from build123d import *

# Parameters (mm, degrees)
SKETCH1_R            = 5.3
BOSS_EXTRUDE1_DEPTH  = 15
M6_CLEARANCE_HOLE1_D = 6.6
BOSS_EXTRUDE3_DEPTH  = 2
BOSS_EXTRUDE2_DEPTH  = 8
SKETCH6_R            = 2.25
CUT_EXTRUDE1_DEPTH   = 27.870888862


with BuildPart() as part:
    # Sketch1 → Boss-Extrude1 (new body, symmetric)
    with BuildSketch(Plane(origin=(0, 0, 0), x_dir=(0, 0, -1), z_dir=(1, 0, 0))):
        Polygon((0, 12.912507763), (-29.037071095, -21.692526033), (-26.738937766, -23.620888862), (-13.883185572, -8.3), (13.883185572, -8.3), (26.738937766, -23.620888862), (29.037071095, -21.692526033), align=None)
        Circle(SKETCH1_R, mode=Mode.SUBTRACT)
    extrude(amount=BOSS_EXTRUDE1_DEPTH, both=True)

    # M6 Clearance Hole1 (through all)
    with Locations(Plane(origin=(0, 3.406774331, 4.060035549), x_dir=(-1, 0, 0), z_dir=(0, -0.64278761, -0.766044443))):
        with Locations((0, -25.282108547)):
            m6_clearance_hole1 = Hole(M6_CLEARANCE_HOLE1_D / 2)

    # Mirror1: M6 Clearance Hole1 across plane
    add(m6_clearance_hole1.mirror(Plane.XY), mode=Mode.SUBTRACT)

    # Sketch7 → Boss-Extrude3 (add)
    with BuildSketch(Plane.ZY.offset(15)):
        with BuildLine():
            Line((-5.150485414, 1.25), (-7.192183257, 1.25))
            ThreePointArc((-7.192183257, 1.25), (7.3, 0), (-7.192183257, -1.25))
            Line((-7.192183257, -1.25), (-5.150485414, -1.25))
            ThreePointArc((-5.150485414, -1.25), (5.3, 0), (-5.150485414, 1.25))
        make_face()
    extrude(amount=BOSS_EXTRUDE3_DEPTH)

    # Sketch5 → Boss-Extrude2 (add)
    with BuildSketch(Plane.ZY.offset(17)):
        with BuildLine():
            Line((-5.150485414, 1.25), (-14.536627571, 1.25))
            Line((-14.536627571, 1.25), (-14.536627571, 3.25))
            Line((-14.536627571, 3.25), (-6.536627571, 3.25))
            ThreePointArc((-6.536627571, 3.25), (7.3, 0), (-6.536627571, -3.25))
            Line((-6.536627571, -3.25), (-6.536627571, -10.25))
            Line((-6.536627571, -10.25), (-14.536627571, -10.25))
            Line((-14.536627571, -10.25), (-14.536627571, -1.25))
            Line((-14.536627571, -1.25), (-5.150485414, -1.25))
            ThreePointArc((-5.150485414, -1.25), (5.3, 0), (-5.150485414, 1.25))
        make_face()
    extrude(amount=BOSS_EXTRUDE2_DEPTH)

    # Sketch6 → Cut-Extrude1 (cut, through all)
    with BuildSketch(Plane(origin=(0, 3.25, 0), x_dir=(1, 0, 0), z_dir=(0, 1, 0))):
        with Locations((-21, 10.536627571)):
            Circle(SKETCH6_R)
    extrude(amount=-CUT_EXTRUDE1_DEPTH, mode=Mode.SUBTRACT)


solid = part.part
CAD build for the part. Positions are in the model's coordinates, mm. A direction names the side the tool comes from. Round coordinates to 2 decimals unless told otherwise and drop trailing zeros. Loops run counter-clockwise (first coordinate to the right, second up) from the corner with the lowest first, then second, coordinate; pieces in that order, holes last.
(1) Drop flat-ended pins along their axis: pin 1 (5 mm diameter, centred on x = -21, z = -10.54, fed in from -Y); pin 2 (4 mm diameter, centred on x = -22.5, z = -12, fed in from +Y); pin 3 (1 mm diameter, centred on x = -19.5, y = 2.5, fed in from -Z). Give the stop position or say it passes through.
(2) Cut at B-B (y = 2). Give the cut face in (x, z), plus the area to 3 significant figures.
(3) Cut at A-A (x = -21). Give the cut face in (y, z), plus the area to 3 significant figures.
(4) Cut at C-C (x = 11). Give the cut face in (y, z).
(5) Cut at D-D (y = 6). Give the cut face in (x, z).
(6) Two-plate mould, pull along X, no slides. Class faces 6 (the cylindrical face through (1.774, -12.851, -19.688)), 7 (the flat face through (-25, -3, -6)), 8 (the flat face through (0.21, -22.643, 27.904)): +X half, -X half, draft (parallel to the pull), parting line (faces both ways), or undercut.
(7) Wall check: line 1 along Y through (x, z) = (-22.5, 0); line 2 along Z through (x, y) = (-21, 2.15); line 3 along X through (y, z) = (-3, -9.5). Give the ranges that are in metal, low to high.
(8) Which spindle directions (+Z, -Z, +X, -X, +Y, -Y) get a long thin tool onto all of the face, cutting with end or side? Do faces 1 (the flat face through (3.543, -16.068, 20.401)), 2 (the flat face through (-21, -6, -14.537)), 3 (the flat face through (-21, 1.25, -8)), 4 (the flat face through (-23, 3.25, -9)), 5 (the flat face through (0, -8.3, 0)). Say none if no direction does.
Findings below:
1. pin 1: stops at y = -10.25
1. pin 2: stops at y = 3.25
1. pin 3: stops at z = -14.54
2. outline: (-25, -14.54) - (-17, -14.54) - (-17, -7.02) - (-15, -7.02) - (-15, -9.16) - (15, -9.16) - (15, -4.91) - (-25, -4.91) - close; (-25, 4.91) - (15, 4.91) - (15, 9.16) - (-15, 9.16) - (-15, 7.02) - (-25, 7.02) - close; hole circle Ø4.5 at (-21, -10.54)
2. area: 341 mm2
3. outline: (-10.25, -14.54) - (-1.25, -14.54) - (-1.25, -12.79) - (-10.25, -12.79) - close; (-10.25, -8.29) - (-1.25, -8.29) - (-1.25, -5.15) arc R5.3 cw (long way) to (1.25, -5.15) - (1.25, -8.29) - (3.25, -8.29) - (3.25, -6.54) arc R7.3 ccw (long way) to (-3.25, -6.54) - (-10.25, -6.54) - close; (1.25, -14.54) - (3.25, -14.54) - (3.25, -12.79) - (1.25, -12.79) - close
3. area: 111 mm2
4. outline: (-23.62, -26.74) - (-21.69, -29.04) - (12.91, 0) - (-21.69, 29.04) - (-23.62, 26.74) - (-8.3, 13.88) - (-8.3, -13.88) - close; hole circle Ø10.6 at (0, 0)
5. outline: (-25, -4.16) - (-15, -4.16) - (-15, -5.8) - (15, -5.8) - (15, 5.8) - (-15, 5.8) - (-15, 4.16) - (-25, 4.16) - close
6. face 6: undercut
6. face 7: -X half
6. face 8: draft
7. line 1: y = -7.3 to -5.3, 5.3 to 7.3
7. line 2: z = -14.54 to -12.79, -8.29 to -4.84, 4.84 to 6.98
7. line 3: x = -25 to -23, -19 to -17, -15 to 15
8. face 1: +X, -X, -Y
8. face 2: -Z, -X, +Y, -Y
8. face 3: -Z, -X
8. face 4: -Z, -X, +Y
8. face 5: +X, -Y
